```python
from build123d import *

# Parameters (mm, degrees)
BOSS_EXTRUDE1_DEPTH = 4.7625
SKETCH2_W           = 25.4
SKETCH2_H           = 31.75
BOSS_EXTRUDE2_DEPTH = 20.6375
SKETCH4_R           = 3.96875
CUT_EXTRUDE2_DEPTH  = 61.241389426
FILLET2_RADIUS      = 15.875
FILLET2_LENGTH      = 25.4
SKETCH5_W           = 11.1125
SKETCH5_H           = 24.885554027
CUT_EXTRUDE3_DEPTH  = 52.587643869
SKETCH6_R           = 3.175
CUT_EXTRUDE4_DEPTH  = 50.416914172
BOSS_EXTRUDE3_START = 1.5875
SKETCH10_W          = 19.05
SKETCH10_H          = 31.75
SKETCH10_R          = 3.175
BOSS_EXTRUDE3_DEPTH = 1.5875
FILLET3_R           = 1.5875


with BuildPart() as part:
    # Sketch1 → Boss-Extrude1 (new body)
    with BuildSketch(Plane(origin=(0, 0, 0), x_dir=(1, 0, 0), z_dir=(0, 1, 0))):
        Polygon((-31.75, 0), (31.75, 0), (31.75, -31.75), (15.875, -31.75), (-15.875, -31.75), (-31.75, -31.75), align=None)
    extrude(amount=BOSS_EXTRUDE1_DEPTH)

    # Sketch2 → Boss-Extrude2 (add)
    with BuildSketch(Plane(origin=(0, 4.7625, 0), x_dir=(1, 0, 0), z_dir=(0, 1, 0))):
        with Locations((0, -15.875)):
            Rectangle(SKETCH2_W, SKETCH2_H)
    extrude(amount=BOSS_EXTRUDE2_DEPTH)

    # Sketch4 → Cut-Extrude2 (cut, through all)
    with BuildSketch(Plane(origin=(12.7, 0, 0), x_dir=(0, 0, -1), z_dir=(1, 0, 0))):
        with Locations((-15.875, 17.78)):
            Circle(SKETCH4_R)
    extrude(amount=-CUT_EXTRUDE2_DEPTH, mode=Mode.SUBTRACT)

    # Fillet2: full round fillet: the end face becomes a half cylinder, R = half its width
    fillet2_face = Plane((0, 25.4, 15.875), x_dir=(1, 0, 0), z_dir=(0, 1, 0))  # on the end face: x along it, z out of the body
    fillet2_slab = fillet2_face.offset(-FILLET2_RADIUS / 2) * Box(FILLET2_LENGTH, 2 * FILLET2_RADIUS, FILLET2_RADIUS, mode=Mode.PRIVATE)  # the body's end, R deep
    fillet2_round = Plane((0, 9.525, 15.875), x_dir=(0, 1, 0), z_dir=(1, 0, 0)) * Cylinder(FILLET2_RADIUS, FILLET2_LENGTH, mode=Mode.PRIVATE)  # its axis R under the face
    add(fillet2_slab - fillet2_round, mode=Mode.SUBTRACT)

    # Sketch5 → Cut-Extrude3 (cut, through all)
    with BuildSketch(Plane.XY.offset(31.75)):
        with Locations((0, 17.205277014)):
            Rectangle(SKETCH5_W, SKETCH5_H)
    extrude(amount=-CUT_EXTRUDE3_DEPTH, mode=Mode.SUBTRACT)

    # Sketch6 → Cut-Extrude4 (cut, through all)
    with BuildSketch(Plane(origin=(0, 4.7625, 0), x_dir=(1, 0, 0), z_dir=(0, 1, 0))):
        with Locations(Location((-20.6375, -7.9375, 0), (0, 0, 270))):
            Circle(SKETCH6_R)
        with Locations(Location((20.6375, -7.9375, 0), (0, 0, 270))):
            Circle(SKETCH6_R)
        with Locations(Location((20.6375, -23.8125, 0), (0, 0, 270))):
            Circle(SKETCH6_R)
        with Locations(Location((-20.6375, -23.8125, 0), (0, 0, 270))):
            Circle(SKETCH6_R)
    extrude(amount=-CUT_EXTRUDE4_DEPTH, mode=Mode.SUBTRACT)

    # Sketch10 → Boss-Extrude3 (add)
    # profile 1 of 2: a face of its own
    with BuildSketch(Plane(origin=(0, 4.7625, 0), x_dir=(1, 0, 0), z_dir=(0, 1, 0)).offset(BOSS_EXTRUDE3_START)):
        with Locations((-22.225, -15.875)):
            Rectangle(SKETCH10_W, SKETCH10_H)
        with Locations(Location((-20.6375, -23.8125, 0), (0, 0, 270))):
            Circle(SKETCH10_R, mode=Mode.SUBTRACT)
        with Locations(Location((-20.6375, -7.9375, 0), (0, 0, 270))):
            Circle(SKETCH10_R, mode=Mode.SUBTRACT)
    # profile 2 of 2: a face of its own
    with BuildSketch(Plane(origin=(0, 4.7625, 0), x_dir=(1, 0, 0), z_dir=(0, 1, 0)).offset(BOSS_EXTRUDE3_START)):
        with Locations((22.225, -15.875)):
            Rectangle(SKETCH10_W, SKETCH10_H)
        with Locations(Location((20.6375, -7.9375, 0), (0, 0, 270))):
            Circle(SKETCH10_R, mode=Mode.SUBTRACT)
        with Locations(Location((20.6375, -23.8125, 0), (0, 0, 270))):
            Circle(SKETCH10_R, mode=Mode.SUBTRACT)
    extrude(amount=-BOSS_EXTRUDE3_DEPTH)

    # Fillet3
    fillet3_edges = [part.edges().sort_by_distance(p)[0] for p in [
        (12.7, 6.35, 15.875),
        (5.55625, 4.7625, 15.875),
        (-5.55625, 4.7625, 15.875),
        (-12.7, 6.35, 15.875),
    ]]
    fillet(fillet3_edges, radius=FILLET3_R)


solid = part.part
```
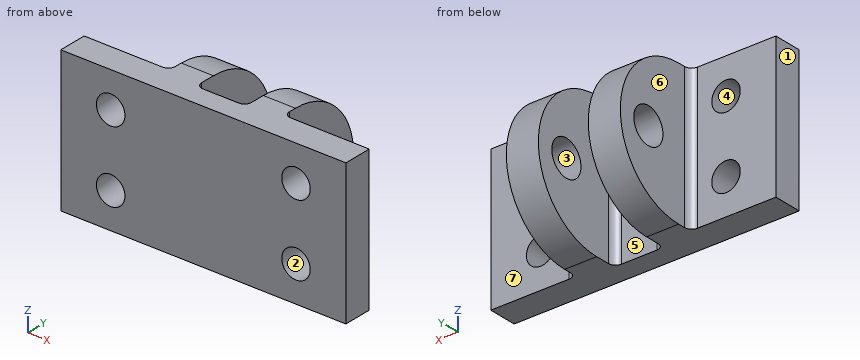
Could you check a few things on this model? Use its own coordinates, in mm. Face numbers are marked on the shaded views. A direction names the side the tool comes from. Round coordinates to 2 decimals unless told otherwise and drop trailing zeros. Write each loop counter-clockwise with the first axis right and the second up, starting at its lowest first coordinate (ties: lowest second). Pieces come first, ordered by that corner, then holes. Notation, with made-up numbers: M -15.75,-29 L 40.25,-29 A23 ccw 40.25,8 Z; hole C 53.25,80 d4. An arc over 180 degrees is marked long. Answer in a Markdown table with one row per item. Add a question column.
Q1. Imagine slicing it at B-B (y = 5.5). Give the number of separate pieces and of enclosed holes in the cut face, then the cut area to 3 significant figures.
Q2. Imagine slicing it at D-D (x = -22). Please give me the cut outline in (y, z), then the cut area to 3 significant figures.
Q3. Will these pins go through, and if not, where does the flat tip stop? pin 1 Ø9.5 at (y, z) = (15, 10) entering from -X; pin 2 Ø8.5 at (y, z) = (17.5, 18) entering from +X; pin 3 Ø6 at (x, z) = (-9.5, 28.5) entering from +Y; pin 4 Ø6.5 at (y, z) = (17.78, 15.875) entering from +X.
Q4. On a 3-axis mill with a long thin cutter (end or side, diameter ignored), from which of +Z, -Z, +X, -X, +Y, -Y can I reach the whole of each face in a straight line? I mean the marked faces 5, 6 and 7. Say none if no direction works.
Q5. If I drill on line 1 (X direction, y = 12.25, z = 6); line 2 (Y direction, x = -15, z = 16); line 3 (X direction, y = 4, z = 6.5), over which ranges is the centre line in solid material (lowest first)? Write a range as from..to.
Q6. If we mould it in two halves opening along X, with no side actions, what happens to the marked faces 1, 2, 3 and 4? For each: +X half, -X half, draft (parallel to the pull), parting line (faces both ways), or undercut.
Values:
| question | item | result |
|---|---|---|
| 1 | separate pieces | 2 |
| 1 | enclosed holes | 4 |
| 1 | area | 1,550 mm^2 |
| 2 | outline | M 0,0 L 6.35,0 L 6.35,5.07 L 0,5.07 Z; M 0,10.81 L 6.35,10.81 L 6.35,20.94 L 0,20.94 Z; M 0,26.68 L 6.35,26.68 L 6.35,31.75 L 0,31.75 Z |
| 2 | area | 129 mm^2 |
| 3 | pin 1 | x = -12.7 |
| 3 | pin 2 | x = 12.7 |
| 3 | pin 3 | y = 22.15 |
| 3 | pin 4 | through |
| 4 | face 5 | +Z, -Z, +Y |
| 4 | face 6 | +Z, -Z, -X, +Y |
| 4 | face 7 | +Z, -Z, +X, +Y |
| 5 | line 1 | -12.7..-5.56, 5.56..12.7 |
| 5 | line 2 | 0..6.35 |
| 5 | line 3 | -31.75..-23.47, -17.81..17.81, 23.47..31.75 |
| 6 | face 1 | -X half |
| 6 | face 2 | undercut |
| 6 | face 3 | draft |
| 6 | face 4 | undercut |
